Can you work these out from the model? Positions are in its coordinate system, mm. Give positions to 0.01 mm unless a question says otherwise; leave off trailing zeros. Order: outer loops, then holes, each group sorted by start corner. A loop starts at its lowest first (then second) coordinate and runs counter-clockwise, first axis right, second up. Notation, with made-up numbers: M 20.5,31 L 40.5,31 A18 ccw 40.5,62 Z; hole C 19,78 d4. An arc over 180 degrees is marked long. Use one line per item in the form item = value. Start each with the question number.
1. Will these pins go through, and if not, where does the flat tip stop? P1, Ø1.1, axis at x = 4, z = 28.5, coming from the -Y side; P2, Ø1.1, axis at x = 4, z = -2.5, coming from the +Y side; P3, Ø4, axis at x = 0, z = 15.5, coming from the +Y side; P4, Ø3.5, axis at x = 0, y = 0, coming from the +Z side.
2. I need wall thicknesses on L1, parallel to X at y = -7.75, z = -52.5; L2, parallel to Y at x = 0, z = 2. Which ranges of each line are inside material? Lowest first, please.
3. I want a section at A-A, the plane x = 0. List the corners of the cut face in (y, z) for me, and give its area (3 significant figures).
Autodesk Inventor part; units mm, degrees
ref_plane "YZ Plane" through (0, 0, 0) normal (1, 0, 0) x (0, 1, 0)
ref_plane "XZ Plane" through (0, 0, 0) normal (0, 1, 0) x (-1, 0, 0)
ref_plane "XY Plane" through (0, 0, 0) normal (0, 0, 1) x (1, 0, 0)
sketch "Sketch1" plane through (0, 0, 0) normal (0, 0, 1) x (1, 0, 0)
  line L0 (0, 3.7) -> (-2.6393, 3.7)
  line L1 (-2.6393, 3.7) -> (-5.5, 6.5607)
  line L2 (-5.5, 6.5607) -> (-5.5, 8.2)
  line L3 (-5.5, 8.2) -> (-3.395, 8.2)
  line L4 (-3.395, 8.2) -> (-3.395, 10)
  line L5 (-3.395, 10) -> (-10, 10)
  line L6 (-10, 10) -> (-10, 3.395)
  line L7 (-10, 3.395) -> (-8.2, 3.395)
  line L8 (-8.2, 3.395) -> (-8.2, 5.5)
  line L9 (-8.2, 5.5) -> (-6.5607, 5.5)
  line L10 (-6.5607, 5.5) -> (-3.7, 2.6393)
  line L11 (-3.7, 2.6393) -> (-3.7, 0)
  line L12 (0, 0) -> (-10, 10) construction
  circle A0 centre (0, 0) radius 2.3
  line L13 (-22.6601, 0) -> (65.9605, 0)
  line L14 (-3.7, 0) -> (0, 0)
  line L15 (0, 0) -> (0, 3.7)
  line L16 (11.2521, 18.9743) -> (53.3004, 18.9743) construction
  line L17 (53.3004, 18.9743) -> (53.3004, -5.624) construction
  line L18 (53.3004, -5.624) -> (11.2521, -5.624) construction
  line L19 (11.2521, -5.624) -> (11.2521, 18.9743) construction
  point P0 (-2.3, 0)
  point P1 (0, 2.3)
  dimension "d0" = 1.5
  dimension "d6" = 6.3
  dimension "d9" = 4.6
  dimension "d18" = 135
  dimension "d22" = 20
  dimension "d34" = 11
  dimension "d35" = 6.79
  dimension "d36" = 1.8
extrude "Extrusion1" add sketch "Sketch1" along normal mid plane 127 contours L15 A0 L13 L11 L10 L9 L8 L7 L6 L5 L4 L3 L2 L1 L0
pattern_circular "Circular Pattern1" count 4 over 360 about axis through (0, 0, -10) along (0, 0, 1) of "Extrusion1"
chamfer "Chamfer1" distance 1.185 angle 45 8 edges at (-3.395, 10, 0) (3.395, 10, 0) (10, 3.395, 0) (10, -3.395, 0) (3.395, -10, 0) (-3.395, -10, 0) (-10, -3.395, 0) (-10, 3.395, 0)
fillet "Fillet1" radius 1.5 4 edges at (-10, 10, 0) (10, 10, 0) (-10, -10, 0) (10, -10, 0)
equation "\"d24\" = Zaxis"
equation "\"GridProcutClearance\" = 3"
equation "\"GridBorderThickness\" = 5"
equation "\"GridBorderFillets\" = 7"
equation "\"GridTotalSize\" = 63"
equation "\"BaseTotalWidth\" = 412"
equation "\"BaseTotalLength\" = 624"
equation "\"DistanceBetweenGrid\" = 5"
equation "\"WorkspaceLength\" = 395"
equation "\"WorkspaceWidth\" = 332"
equation "\"AxesBaseFillet\" = 15"
equation "\"Zaxis\" = 127"
properties part number "2020aluminum_extrusion_black" material "Aluminum 6061"
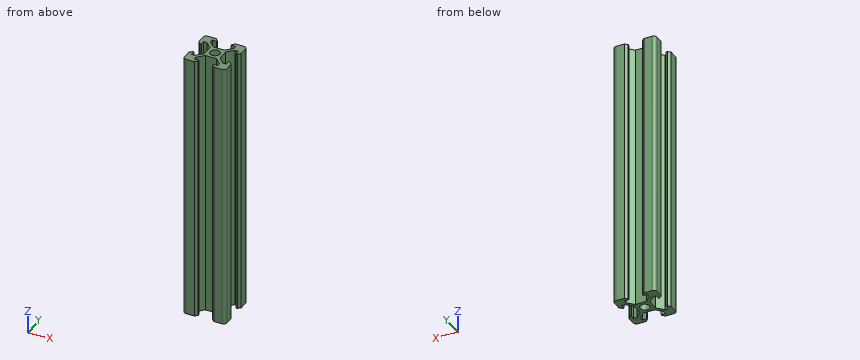
Check result:
q1.P1 = -9.97
q1.P2 = 9.97
q1.P3 = 3.7
q1.P4 = through
q2.L1 = -10 to -5.5, 5.5 to 10
q2.L2 = -3.7 to -2.3, 2.3 to 3.7
q3.outline = M -3.7,-63.5 L -2.3,-63.5 L -2.3,63.5 L -3.7,63.5 Z; M 2.3,-63.5 L 3.7,-63.5 L 3.7,63.5 L 2.3,63.5 Z
q3.area = 356 mm2
